Design review of the part built by this model. Coordinates are the model's own, in mm. A direction names the side the tool comes from. Round coordinates to 2 decimals unless told otherwise and drop trailing zeros. Order: outer loops, then holes, each group sorted by start corner. A loop starts at its lowest first (then second) coordinate and runs counter-clockwise, first axis right, second up. Notation, with made-up numbers: (4.5, 23.25) - (37.5, 23.25) arc R27 cw to (37.5, 55.25) - close; hole circle Ø11 at (50, 35.5). An arc over 180 degrees is marked (long way). Write item = value, one per line.
from build123d import *

# Parameters (mm, degrees)
F0_W     = 393.7
F0_H     = 304.8
F1_DEPTH = 19.05
F2_W     = 333.375
F2_H     = 266.7
F3_DEPTH = 558.8
F4_W     = 307.975
F4_H     = 533.4
F5_DEPTH = 247.65
F6_W     = 307.975
F6_H     = 533.4
F7_DEPTH = 6.35


with BuildPart() as f1:
    # F0 (on Front) → F1 (new body)
    with BuildSketch(Plane.XZ):
        Rectangle(F0_W, F0_H)
    extrude(amount=F1_DEPTH)

    # F2 (on face) → F3 (join)
    with BuildSketch(Plane(origin=(0, 0, 0), x_dir=(-1, 0, 0), z_dir=(0, 1, 0))):
        Rectangle(F2_W, F2_H)
    extrude(amount=F3_DEPTH)

    # F4 (on face) → F5 (cut)
    with BuildSketch(Plane.XY.offset(133.35)):
        with Locations((0, 279.4)):
            Rectangle(F4_W, F4_H)
    extrude(amount=-F5_DEPTH, mode=Mode.SUBTRACT)

    # F6 (on face) → F7 (cut)
    with BuildSketch(Plane(origin=(0, 0, -133.35), x_dir=(1, 0, 0), z_dir=(0, 0, -1))):
        with Locations((0, -279.4)):
            Rectangle(F6_W, F6_H)
    extrude(amount=-F7_DEPTH, mode=Mode.SUBTRACT)


solid = f1.part
1) To check wall thickness, follow L1, parallel to Y at x = 76, z = -82; L2, parallel to X at y = 59.5, z = -73; L3, parallel to Z at x = 93, y = 125. State the ranges of each line that lie inside material, in increasing order. Write a range as from..to.
Findings:
L1 = -19.05..12.7, 546.1..558.8
L2 = -166.69..-153.99, 153.99..166.69
L3 = -127..-114.3
2) We need section C-C on x = -23.5. Write out the cut boundary in (y, z).
Findings:
outline = (-19.05, -152.4) - (0, -152.4) - (0, -133.35) - (12.7, -133.35) - (12.7, -127) - (546.1, -127) - (546.1, -133.35) - (558.8, -133.35) - (558.8, 133.35) - (546.1, 133.35) - (546.1, -114.3) - (12.7, -114.3) - (12.7, 133.35) - (0, 133.35) - (0, 152.4) - (-19.05, 152.4) - close
3) Clearance check with flat-ended pins moving along their axes: pin 1 Ø4 at (y, z) = (174, -10.5) entering from +X; pin 2 Ø12 at (y, z) = (245.5, -13) entering from -X; pin 3 Ø5 at (x, y) = (87.5, 183) entering from -Z. State where each tip first meets the part, or that it passes through.
Findings:
pin_1 = 166.69
pin_2 = -166.69
pin_3 = -127
4) We need section A-A on y = 130.5. Write out the cut boundary in (x, z).
Findings:
outline = (-166.69, -133.35) - (-153.99, -133.35) - (-153.99, -127) - (153.99, -127) - (153.99, -133.35) - (166.69, -133.35) - (166.69, 133.35) - (153.99, 133.35) - (153.99, -114.3) - (-153.99, -114.3) - (-153.99, 133.35) - (-166.69, 133.35) - close
5) For faces 4 (the flat face through (-2, 12.7, 11)), 5 (the flat face through (166.688, 275, -2)), 6 (the flat face through (161, 278, 133.35)), 7 (the flat face through (-166.688, 275, -2)), 8 (the flat face through (-196.85, -9, -2)), list the 3-axis set-ups (+Z, -Z, +X, -X, +Y, -Y) from which the entire face can be reached by the end or side of a thin tool; tool diameter is ignored.
Findings:
face_4 = +Z
face_5 = +Z, -Z, +X, +Y
face_6 = +Z, +X, -X, +Y
face_7 = +Z, -Z, -X, +Y
face_8 = +Z, -Z, -X, +Y, -Y
6) We need section B-B on z = -6. Write out the cut boundary in (x, y).
Findings:
outline = (-196.85, -19.05) - (196.85, -19.05) - (196.85, 0) - (166.69, 0) - (166.69, 558.8) - (-166.69, 558.8) - (-166.69, 0) - (-196.85, 0) - close; hole (-153.99, 12.7) - (153.99, 12.7) - (153.99, 546.1) - (-153.99, 546.1) - close
7) The part is to be moulded in two halves that separate along Y. For faces 1 (the flat face through (-2, 276, -127)), 2 (the flat face through (161, 278, -133.35)), 3 (the flat face through (-3, -19.05, 2)), say which applies: released by +Y, released by -Y, zero draft, split by the parting line, or undercut.
Findings:
face_1 = undercut
face_2 = zero draft
face_3 = released by -Y
